Source: CAD feature listing. Evaluate the final solid. Frame: model axes, mm. Face numbers are marked on the shaded views. A direction names the side the tool comes from. Give positions to 0.01 mm unless a question says otherwise; leave off trailing zeros. Put each result on its own line as item: value.
```python
from build123d import *

# Parameters (mm, degrees)
BOSS_EXTRUDE1_DEPTH      = 50
BOSS_EXTRUDE1_DEPTH_BACK = 50
SKETCH2_W                = 80
SKETCH2_H                = 150
CUT_EXTRUDE1_DEPTH       = 367.509355196
SKETCH3_R                = 45
BOSS_EXTRUDE2_DEPTH      = 10
FILLET1_R                = 5


with BuildPart() as part:
    # Sketch1 → Boss-Extrude1 (new, two sides: drawn at the far end of the back side and taken through both)
    with BuildSketch(Plane.XY.offset(-BOSS_EXTRUDE1_DEPTH_BACK)):
        with BuildLine():
            Line((-49, 0), (49, 0))
            Line((49, 0), (48.785008207, -245.999906054))
            Line((48.785008207, -245.999906054), (40.709882529, -313.518735615))
            ThreePointArc((40.709882529, -313.518735615), (0, -349.649909839), (-40.709882529, -313.518735615))
            Line((-40.709882529, -313.518735615), (-48.785008207, -245.999906054))
            Line((-48.785008207, -245.999906054), (-49, 0))
        make_face()
    extrude(amount=BOSS_EXTRUDE1_DEPTH + BOSS_EXTRUDE1_DEPTH_BACK)

    # Sketch2 → Cut-Extrude1 (cut, through all)
    with BuildSketch(Plane(origin=(48.999962574, -0.042823552, 0), x_dir=(0, 0, -1), z_dir=(0.9999996181052956, -0.0008739503779168433, 0))):
        with Locations((0, -274.649791967)):
            Rectangle(SKETCH2_W, SKETCH2_H)
    extrude(amount=-CUT_EXTRUDE1_DEPTH, mode=Mode.SUBTRACT)

    # Sketch3 → Boss-Extrude2 (add)
    with BuildSketch(Plane(origin=(0, 0, 0), x_dir=(1, 0, 0), z_dir=(0, 1, 0))):
        with Locations(Location((0, 0, 0), (0, 0, 270))):
            Circle(SKETCH3_R)
    extrude(amount=BOSS_EXTRUDE2_DEPTH)

    # Fillet1
    fillet1_edges = [part.edges().sort_by_distance(p)[0] for p in [
        (0, 0, -45),
    ]]
    fillet(fillet1_edges, radius=FILLET1_R - 0.0001)  # a hair under: the kernel refuses the full size


with BuildPart() as part_1:
    # Body-Move/Copy1: moved
    add(part.part.moved(Location((0, 308.649909839, 0))))


solid = part_1.part
```
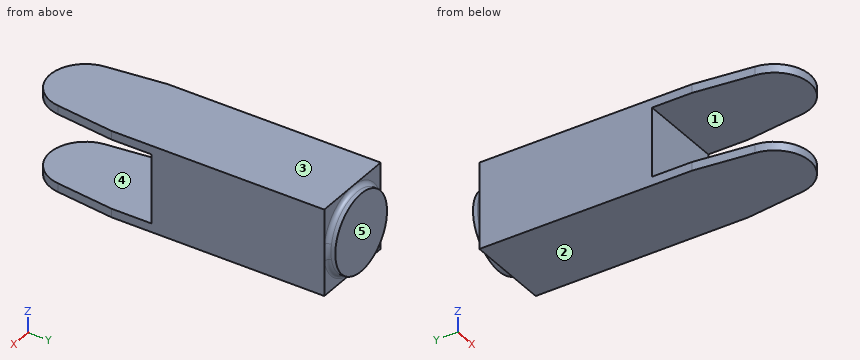
1) Pin query (flat end, axial travel): P1, Ø10, axis at x = -17.5, z = -21, coming from the -Y side. Return the tip coordinate at first contact, or that it passes through.
Check result:
P1: y = 109.01
2) Access query for the marked faces 4 and 5. Directions: +Z, -Z, +X, -X, +Y, -Y. A direction counts if a zero-diameter tool reaches every point of the face in a straight line with its end or side. Return the directions, or none.
Check result:
face 4: +X, -X, -Y
face 5: +Z, -Z, +X, -X, +Y
3) Material intervals for line 1 along Z through (x, y) = (39, 7); line 2 along Y through (x, z) = (-4, 36); line 3 along X through (y, z) = (236, 46), sorted ascending. Write a range as [from, to].
Check result:
line 1: [-50, -40], [40, 50]
line 2: [109, 318.65]
line 3: [-48.94, 48.94]
4) Mould query, pull axis Z, two halves, no side actions, for the marked faces 1, 2 and 3. Classes: pulls with the +Z half, pulls with the -Z half, needs draft (parallel to the pull), parting line crosses it, or undercut.
Check result:
face 1: undercut
face 2: pulls with the -Z half
face 3: pulls with the +Z half
